Can you work these out from the model? Positions are in its coordinate system, mm. A direction names the side the tool comes from. Round coordinates to 2 decimals unless told otherwise and drop trailing zeros. Write each loop counter-clockwise with the first axis right and the second up, starting at its lowest first coordinate (ties: lowest second). Pieces come first, ordered by that corner, then holes.
Q1. If we section it at A-A (z = 26.5): Please give me the cut outline in (x, y) (3 decimals), plus the area to 3 significant figures.
Q2. For faces 1 (the flat face through (2, -3, 0)), 2 (the flat face through (2.072, 1.174, -4.785)), 3 (the flat face through (0, 0, 38.1)), which set-ups out of +Z, -Z, +X, -X, +Y, -Y let a thin tool reach every point of the face, with its end or its side?
Q3. I'm going to push flat-ended pins straight in: pin 1 Ø5 at (x, z) = (1.5, 26.5) entering from -Y (3 decimals); pin 2 Ø2 at (y, z) = (-1, 12.5) entering from +X (3 decimals); pin 3 Ø1 at (y, z) = (-2, 13) entering from +X. Where does each tip first touch, or does it pass through?
Q4. We'd pull the mould along Y, two halves only. Please class faces 4 (the flat face through (0, 0, -3.175)), 5 (the flat face through (-2, -2, -6.35)), 6 (the cylindrical face through (-0.69, 3.1, 18.53)): +Y half, -Y half, draft (parallel to the pull), parting line (faces both ways), or undercut.
Q5. Please list where these lines run through material, in increasing order: line 1 along X through (y, z) = (-0.25, 4); line 2 along Z through (x, y) = (1, 0.25) (3 decimals).
Autodesk Inventor part; units mm, degrees
ref_plane "YZ Plane" through (0, 0, 0) normal (1, 0, 0) x (0, 1, 0)
ref_plane "XZ Plane" through (0, 0, 0) normal (0, 1, 0) x (-1, 0, 0)
ref_plane "XY Plane" through (0, 0, 0) normal (0, 0, 1) x (1, 0, 0)
sketch "Sketch1" plane through (0, 0, 0) normal (0, 0, 1) x (1, 0, 0)
  circle A0 centre (0, 0) radius 3.175
  dimension "d0" = 6.35
extrude "Extrusion1" add sketch "Sketch1" along normal blind 38.1
sketch "Sketch2" plane through (0, 0, 0) normal (0, 0, -1) x (-1, 0, 0)
  circle A0 centre (0, 0) radius 3.175
  circle A1 centre (0, 0) radius 4.7625
  dimension "d3" = 9.525
extrude "Extrusion2" add sketch "Sketch2" along normal blind 6.35 contours A0 | A1
sketch "Sketch3" plane through (0, 0, -6.35) normal (0, 0, -1) x (-1, 0, 0)
  circle A0 centre (0, 0) radius 4.7625
  line L0 (-1.3748, 2.3812) -> (1.3748, 2.3813)
  line L1 (1.3748, 2.3813) -> (2.7496, 0)
  line L2 (2.7496, 0) -> (1.3748, -2.3812)
  line L3 (1.3748, -2.3812) -> (-1.3748, -2.3812)
  line L4 (-1.3748, -2.3812) -> (-2.7496, 0)
  line L5 (-2.7496, 0) -> (-1.3748, 2.3812)
  dimension "d6" = 4.7625
extrude "Extrusion3" cut sketch "Sketch3" against normal blind 3.175 contours L0 L1 L2 L3 L4 L5
chamfer "Chamfer1" distance 0.508 angle 45 3 edges at (-3.175, 0, 38.1) (4.7625, 0, 0) (4.7625, 0, -6.35)
thread "Thread1"
properties part number "14-20 x750" material "Steel"
A:
1. outline: circle Ø6.35 at (0, 0)
1. area: 31.7 mm2
2. face 1: +Z
2. face 2: -Z
2. face 3: +Z, +X, -X, +Y, -Y
3. pin 1: stops at y = -3.175
3. pin 2: stops at x = 3.175
3. pin 3: stops at x = 2.8
4. face 4: undercut
4. face 5: draft
4. face 6: parting line
5. line 1: x = -3.17 to 3.17
5. line 2: z = -3.175 to 38.1
